For this review, take the finished solid that the model builds, in its own axes (mm). Coordinates: 2 decimals unless noted, no trailing zeros. Loops run counter-clockwise (first coordinate to the right, second up) from the corner with the lowest first, then second, coordinate; pieces in that order, holes last. Notation, with made-up numbers: (1.5, 55) -> (16.5, 55) arc R9 cw to (16.5, 67) -> close; hole circle Ø9 at (-21.75, -31). An arc over 180 degrees is marked (long way). Use a Markdown table: item, result.
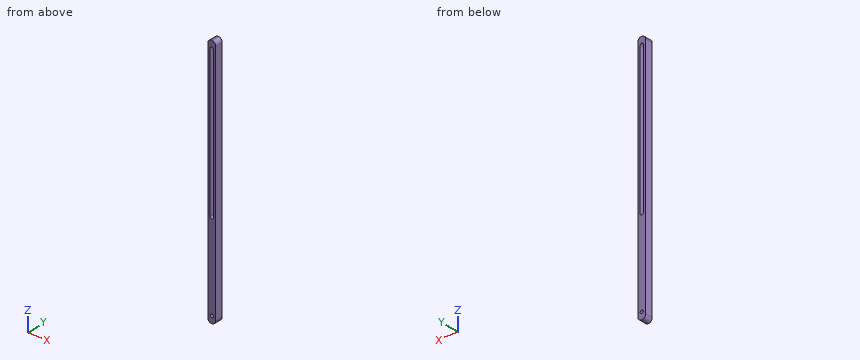
from build123d import *

# Parameters (mm, degrees)
F0_W     = 25
F0_H     = 800
F1_DEPTH = 25
F2_W     = 10
F2_H     = 475
F3_DEPTH = 25
F4_R     = 5
F5_DEPTH = 25
F7_DEPTH = 25
F9_DEPTH = 25
F10_R    = 12.49999
F11_R    = 12.49999


# Not quite as in the source:
# - a fillet or chamfer is up to 0.001 mm smaller than in the source, because OpenCascade refuses the exact size


with BuildPart() as f1:
    # F0 (on Front) → F1 (new body)
    with BuildSketch(Plane.XZ):
        Rectangle(F0_W, F0_H)
    extrude(amount=F1_DEPTH)

    # F2 (on face) → F3 (cut)
    with BuildSketch(Plane.XZ.offset(25)):
        with Locations((0, 138.0000114441)):
            Rectangle(F2_W, F2_H)
    extrude(amount=-F3_DEPTH, mode=Mode.SUBTRACT)

    # F4 (on face) → F5 (cut)
    with BuildSketch(Plane.XZ.offset(25)):
        with Locations((0, -377.3987293243)):
            Circle(F4_R)
    extrude(amount=-F5_DEPTH, mode=Mode.SUBTRACT)

    # F6 (on face) → F7 (cut)
    with BuildSketch(Plane.XZ.offset(25)):
        with BuildLine():
            Line((-5, 375.5000114441), (5, 375.5000114441))
            ThreePointArc((5, 375.5000114441), (0, 380.5000114441), (-5, 375.5000114441))
        make_face()
    extrude(amount=-F7_DEPTH, mode=Mode.SUBTRACT)

    # F8 (on face) → F9 (cut)
    with BuildSketch(Plane.XZ.offset(25)):
        with BuildLine():
            Line((5, -99.4999885559), (-5, -99.4999885559))
            ThreePointArc((-5, -99.4999885559), (0, -104.4999885559), (5, -99.4999885559))
        make_face()
    extrude(amount=-F9_DEPTH, mode=Mode.SUBTRACT)

    # F10 (radius 12.5 in the source; OpenCascade refuses exactly that, so slightly less here)
    f10_edges = [f1.edges().sort_by_distance(p)[0] for p in [
        (-12.5, -12.5, 400),
        (12.5, -12.5, 400),
    ]]
    fillet(f10_edges, radius=F10_R)

    # F11 (radius 12.5 in the source; OpenCascade refuses exactly that, so slightly less here)
    f11_edges = [f1.edges().sort_by_distance(p)[0] for p in [
        (-12.5, -12.5, -400),
        (12.5, -12.5, -400),
    ]]
    fillet(f11_edges, radius=F11_R)


solid = f1.part
(1) For line 1 along X through (y, z) = (-4.75, 36); line 2 along Z through (x, y) = (-4, -18.25); line 3 along Z through (x, y) = (2.75, -10.25), list the stretches that pass through material, from the lowest coordinate up.
Found:
| item | result |
|---|---|
| line 1 | x = -12.5 to -5, 5 to 12.5 |
| line 2 | z = -399.34 to -380.4, -374.4 to -102.5, 378.5 to 399.34 |
| line 3 | z = -399.69 to -381.57, -373.22 to -103.68, 379.68 to 399.69 |
(2) Take a section at A-A on z = 190.5. Write out the cut boundary in (x, y), plus the area to 3 significant figures.
Found:
| item | result |
|---|---|
| outline | (-12.5, -25) -> (-5, -25) -> (-5, 0) -> (-12.5, 0) -> close; (5, -25) -> (12.5, -25) -> (12.5, 0) -> (5, 0) -> close |
| area | 375 mm^2 |
(3) For pin 1 Ø1 at (x, y) = (-4, -19) entering from +Z; pin 2 Ø10 at (x, y) = (9, -15) entering from -Z; pin 3 Ø1.5 at (x, y) = (9.5, -9) entering from -Z, all flat-tipped, find the tip position at first contact; note any pin that passes through.
Found:
| item | result |
|---|---|
| pin 1 | stops at z = 399.5 |
| pin 2 | stops at z = -399.34 |
| pin 3 | stops at z = -396.43 |
(4) Take a section at B-B on y = -19.75. State how many separate pieces and enclosed holes the cut face has, plus the area to 3 significant figures.
Found:
| item | result |
|---|---|
| separate pieces | 1 |
| enclosed holes | 2 |
| area | 15,000 mm^2 |
